from build123d import *

# Parameters (mm, degrees)
F0_W     = 76.2
F0_H     = 21.59
F1_DEPTH = 2.54
F2_W     = 2.54
F2_H     = 21.59
F3_DEPTH = 10.16
F5_DEPTH = 25.4
F7_DEPTH = 21.59


# Not quite as in the source:
# - a feature names something its author has since deleted; it is built from what else it names


with BuildPart() as f1:
    # F0 (on Top) → F1 (new body)
    with BuildSketch(Plane.XY):
        with Locations((38.1, 10.795)):
            Rectangle(F0_W, F0_H)
    extrude(amount=F1_DEPTH)

    # F2 (on face) → F3 (join)
    with BuildSketch(Plane.XY.offset(2.54)):
        with Locations((1.27, 10.795)):
            Rectangle(F2_W, F2_H)
        with Locations((74.93, 10.795)):
            Rectangle(F2_W, F2_H)
    extrude(amount=F3_DEPTH)

    # F4 (on face) → F5 (cut)
    with BuildSketch(Plane.XY.offset(2.54)):
        with BuildLine():
            ThreePointArc((29.21, 21.59), (38.1, 12.7), (46.99, 21.59))
            Line((46.99, 21.59), (29.21, 21.59))
        make_face()
        with BuildLine():
            Line((29.21, 21.59), (46.99, 21.59))
            ThreePointArc((46.99, 21.59), (38.1, 30.48), (29.21, 21.59))
        make_face()
    extrude(amount=-F5_DEPTH, mode=Mode.SUBTRACT)

    # F6 (on face) → F7 (join, through all)
    with BuildSketch(Plane.XZ):
        Polygon((0, 8.89), (0, 12.7), (-1.27, 12.7), align=None)
        Polygon((76.2, 12.7), (76.2, 8.89), (77.47, 12.7), align=None)
    extrude(amount=-F7_DEPTH)


solid = f1.part
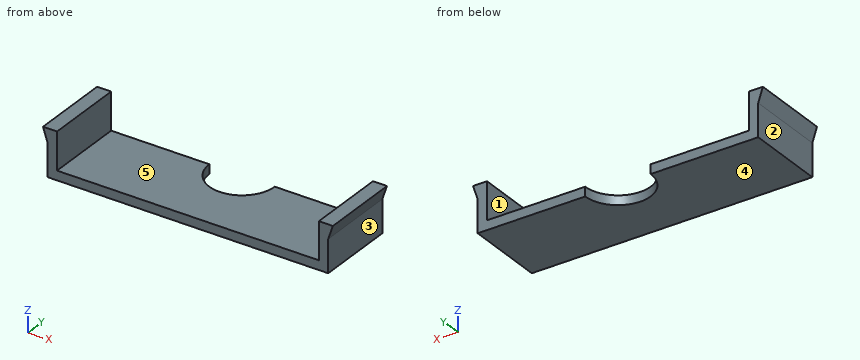
Can you work these out from the model? Positions are in its coordinate system, mm. Face numbers are marked on the shaded views. A direction names the side the tool comes from. Round coordinates to 2 decimals unless told otherwise and drop trailing zeros. Order: outer loops, then holes, each group sorted by start corner. A loop starts at its lowest first (then second) coordinate and runs counter-clockwise, first axis right, second up. Notation, with made-up numbers: M 68,-6 L 96,-6 A18 ccw 96,9 Z; hole C 78.5,15 d9. An arc over 180 degrees is marked long. Use a Markdown table: item, result.
1) Imagine slicing it at A-A (y = 16.5). List the corners of the cut face in (x, z) for me, then the cut area to 3 significant figures.
Geometry says:
| item | result |
|---|---|
| outline | M -1.27,12.7 L 0,8.89 L 0,0 L 30.81,0 L 30.81,2.54 L 2.54,2.54 L 2.54,12.7 Z; M 45.39,0 L 76.2,0 L 76.2,8.89 L 77.47,12.7 L 73.66,12.7 L 73.66,2.54 L 45.39,2.54 Z |
| area | 213 mm² |
2) Imagine slicing it at C-C (y = 9.5). List the corners of the cut face in (x, z) for me.
Geometry says:
| item | result |
|---|---|
| outline | M -1.27,12.7 L 0,8.89 L 0,0 L 76.2,0 L 76.2,8.89 L 77.47,12.7 L 73.66,12.7 L 73.66,2.54 L 2.54,2.54 L 2.54,12.7 Z |
3) I'm going to push flat-ended pins straight in: P1, Ø4, axis at x = 62, y = 10.5, coming from the +Z side; P2, Ø2, axis at y = 17.5, z = 9.5, coming from the +X side; P3, Ø3, axis at y = 12, z = 7.5, coming from the -X side. Where does each tip first touch, or does it pass through?
Geometry says:
| item | result |
|---|---|
| P1 | stops at z = 2.54 |
| P2 | stops at x = 76.74 |
| P3 | stops at x = -0.04 |
4) On a 3-axis mill with a long thin cutter (end or side, diameter ignored), from which of +Z, -Z, +X, -X, +Y, -Y can I reach the whole of each face in a straight line? I mean the marked faces 4 and 5. Say none if no direction works.
Geometry says:
| item | result |
|---|---|
| face 4 | -Z, +X, -X, +Y, -Y |
| face 5 | +Z, +Y, -Y |
5) Imagine slicing it at D-D (x = 38.1). List the corners of the cut face in (y, z) for me.
Geometry says:
| item | result |
|---|---|
| outline | M 0,0 L 12.7,0 L 12.7,2.54 L 0,2.54 Z |
6) If we mould it in two halves opening along X, with no side actions, what happens to the marked faces 1, 2 and 3? For each: +X half, -X half, draft (parallel to the pull), parting line (faces both ways), or undercut.
Geometry says:
| item | result |
|---|---|
| face 1 | undercut |
| face 2 | -X half |
| face 3 | +X half |
7) Imagine slicing it at B-B (z = 9.75). List the corners of the cut face in (x, y) for me.
Geometry says:
| item | result |
|---|---|
| outline | M -0.29,0 L 2.54,0 L 2.54,21.59 L -0.29,21.59 Z; M 73.66,0 L 76.49,0 L 76.49,21.59 L 73.66,21.59 Z |
8) If I drill on line 1 along X through (y, z) = (12.5, 6.5); line 2 along Z through (x, y) = (48, 12); line 3 along X through (y, z) = (12, 0.5), over which ranges is the centre line in solid material (lowest first)?
Geometry says:
| item | result |
|---|---|
| line 1 | x = 0 to 2.54, 73.66 to 76.2 |
| line 2 | z = 0 to 2.54 |
| line 3 | x = 0 to 76.2 |
